Design review of the part built by this model. Coordinates are the model's own, in mm. Face numbers are marked on the shaded views. Coordinates: 2 decimals unless noted, no trailing zeros. Loops run counter-clockwise (first coordinate to the right, second up) from the corner with the lowest first, then second, coordinate; pieces in that order, holes last.
Q1. Draft analysis for pull direction X (two halves, no side actions). For the marked faces 1, 2 and 3, state which applies: released by +X, released by -X, zero draft, split by the parting line, or undercut.
Q2. Wall thickness on probe 1 along X at (y, z) = (0.1, 9.75); probe 2 along Y at (x, z) = (0, 11.95); probe 3 along Y at (x, z) = (0, 12.05): over which ranges is each line inside the solid? List them lowest first.
Q3. Add section D-D on y = 1.35. Give the boundary of the cut face in (x, z).
Q4. For P1, Ø3, axis at x = 1, y = 0, coming from the -Z side; P2, Ø1, axis at x = 0, y = 0, coming from the +Z side; P3, Ø3, axis at y = 1, z = 3.5, coming from the -X side; P4, Ø1.5, axis at x = 0, z = 3.5, coming from the +Y side, all flat-tipped, find the tip position at first contact; note any pin that passes through.
Q5. Add section C-C on z = 9.5. Give the boundary of the cut face in (x, y).
Q6. Add section A-A on y = 0. Give the boundary of the cut face in (x, z).
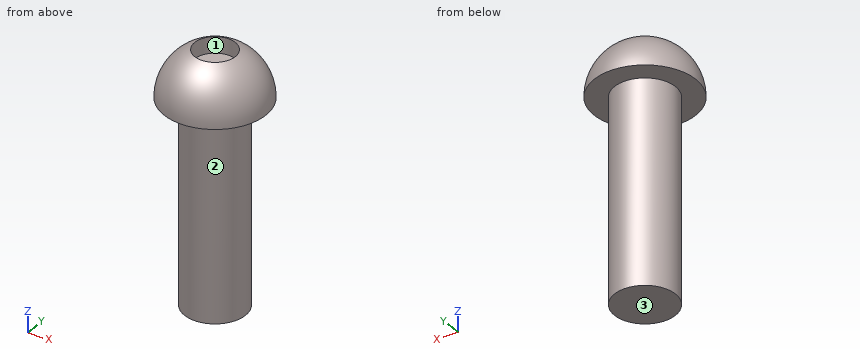
Autodesk Inventor part; units mm, degrees
ref_plane "Work Plane1" through (0, 0, 12.5079) normal (0, 0, 1) x (1, 0, 0)
ref_plane "YZ Plane" through (0, 0, 0) normal (1, 0, 0) x (0, 1, 0)
ref_plane "XZ Plane" through (0, 0, 0) normal (0, 1, 0) x (-1, 0, 0)
sketch "Sketch1" plane through (0, 0, 0) normal (0, 0, 1) x (1, 0, 0)
  circle A0 centre (0, 0) radius 1.5
  dimension "d0" = 3
extrude "Extrusion1" add sketch "Sketch1" along normal blind 10
sketch "Sketch2" plane through (0, 0, 0) normal (0, 1, 0) x (-1, 0, 0)
  line L0 (1.5, 10) -> (-1.5, 10)
  line L1 (1.5, 0) -> (-1.5, 0)
  line L2 (1.5, 10) -> (-1.5, 10)
  line L3 (0, 12.0549) -> (0, 7.9451)
  arc A0 (2.5079, 10) -> (-2.5079, 10) centre (0, 10) ccw
  line L4 (-2.5079, 10) -> (2.5079, 10)
  line L5 (0, 10) -> (0, 12.5079)
  point P0 (0, 0)
revolve "Revolution1" add sketch "Sketch2" angle 360 about axis through (0, 0, 12.0549) along (0, 0, -1) picked at (0.5212, 11.3386) contours L0 L3 L5 A0 L4
ref_plane "Work Plane1" through (0, 0, 12.5079) normal (0, 0, 1) x (1, 0, 0)
sketch "Sketch3" plane through (0, 0, 12.5079) normal (0, 0, 1) x (1, 0, 0)
  circle A0 centre (0, 0) radius 1
  dimension "d4" = 2
extrude "Extrusion2" cut sketch "Sketch3" against normal blind 1
properties part number "Perno"
Entries:
1. face 1: undercut
1. face 2: split by the parting line
1. face 3: zero draft
2. probe 1: x = -1.5 to 1.5
2. probe 2: y = -1.58 to -1, 1 to 1.58
2. probe 3: y = -1.44 to -1, 1 to 1.44
3. outline: (-2.11, 10) - (-0.65, 10) - (-0.65, 0) - (0.65, 0) - (0.65, 10) - (2.11, 10) arc R2.11 ccw to start
4. P1: stops at z = 0
4. P2: stops at z = 11.51
4. P3: stops at x = -1.5
4. P4: stops at y = 1.5
5. outline: circle Ø3 at (0, 0)
6. outline: (-2.51, 10) - (-1.5, 10) - (-1.5, 0) - (1.5, 0) - (1.5, 10) - (2.51, 10) arc R2.51 ccw to (1, 12.3) - (1, 11.51) - (-1, 11.51) - (-1, 12.3) arc R2.51 ccw to start
